Read the model definition and answer for the solid it produces. Units are mm, in the model's axes. Face numbers are marked on the shaded views. Round coordinates to 2 decimals unless told otherwise and drop trailing zeros. Write each loop counter-clockwise with the first axis right and the second up, starting at its lowest first coordinate (ties: lowest second). Pieces come first, ordered by that corner, then holes. Notation, with made-up numbers: (33.5, 29.5) -> (39.5, 29.5) arc R19 cw to (39.5, 45.5) -> close; hole circle Ø5 at (48, 27.5). An arc over 180 degrees is marked (long way). Return JSON: item names as keys, results as strings.
from build123d import *

# Parameters (mm, degrees)
BOSS_EXTRUDE1_DEPTH = 6.35
SKETCH2_W           = 18
SKETCH2_H           = 6.35
CUT_EXTRUDE1_DEPTH  = 148.509567486
SKETCH4_W           = 60
SKETCH4_H           = 105
CUT_EXTRUDE2_DEPTH  = 3.1
SKETCH5_R           = 1.6
CUT_EXTRUDE3_DEPTH  = 148.509567486


with BuildPart() as part:
    # Sketch1 → Boss-Extrude1 (new body)
    with BuildSketch(Plane(origin=(0, 0, 0), x_dir=(1, 0, 0), z_dir=(0, 1, 0))):
        Polygon((64.951905284, 87.5), (-64.951905284, 87.5), (-108.253175473, 12.5), (-43.301270189, -100), (43.301270189, -100), (108.253175473, 12.5), align=None)
    extrude(amount=BOSS_EXTRUDE1_DEPTH)

    # Sketch2 → Cut-Extrude1 (cut, through all)
    with BuildSketch(Plane(origin=(0, 6.35, 0), x_dir=(1, 0, 0), z_dir=(0, 1, 0))):
        with Locations((-29, -90.525)):
            Rectangle(SKETCH2_W, SKETCH2_H)
        with Locations((29, -90.525)):
            Rectangle(SKETCH2_W, SKETCH2_H)
        Polygon((-62.146580335, 79.758965344), (-56.647319021, 76.583965344), (-65.647319021, 60.995508076), (-71.146580335, 64.170508076), align=None)
        Polygon((-94.647319021, 10.766034656), (-85.647319021, 26.354491924), (-91.146580335, 29.529491924), (-100.146580335, 13.941034656), align=None)
        Polygon((100.146580335, 13.941034656), (91.146580335, 29.529491924), (85.647319021, 26.354491924), (94.647319021, 10.766034656), align=None)
        Polygon((56.647319021, 76.583965344), (62.146580335, 79.758965344), (71.146580335, 64.170508076), (65.647319021, 60.995508076), align=None)
    extrude(amount=-CUT_EXTRUDE1_DEPTH, mode=Mode.SUBTRACT)

    # Sketch4 → Cut-Extrude2 (cut)
    with BuildSketch(Plane(origin=(0, 6.35, 0), x_dir=(1, 0, 0), z_dir=(0, 1, 0))):
        Rectangle(SKETCH4_W, SKETCH4_H)
    extrude(amount=-CUT_EXTRUDE2_DEPTH, mode=Mode.SUBTRACT)

    # Sketch5 → Cut-Extrude3 (cut, through all)
    with BuildSketch(Plane(origin=(0, 6.35, 0), x_dir=(1, 0, 0), z_dir=(0, 1, 0))):
        with Locations(Location((0, 72.5, 0), (0, 0, 270))):
            Circle(SKETCH5_R)
        with Locations(Location((-62.786841774, -36.25, 0), (0, 0, 270))):
            Circle(SKETCH5_R)
        with Locations(Location((62.786841774, -36.25, 0), (0, 0, 270))):
            Circle(SKETCH5_R)
    extrude(amount=-CUT_EXTRUDE3_DEPTH, mode=Mode.SUBTRACT)


solid = part.part
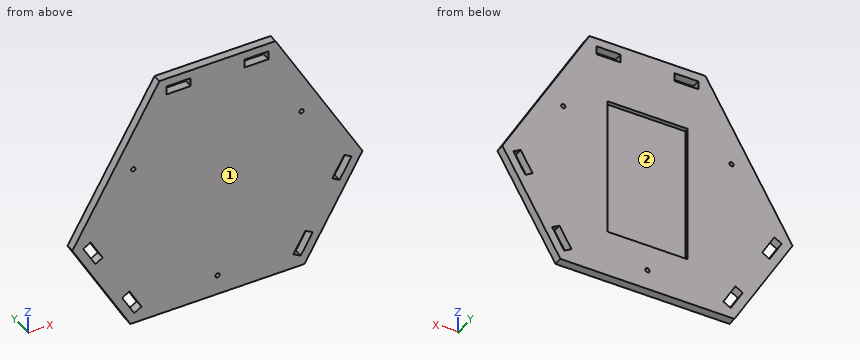
Item 1: Section C-C (z = 49) is taken. Give the vertices of the cut face in (x, y), then the cut area to 3 significant figures.
Worked answers:
{"outline": "(-72.75, 0) -> (72.75, 0) -> (72.75, 6.35) -> (30, 6.35) -> (30, 3.25) -> (-30, 3.25) -> (-30, 6.35) -> (-72.75, 6.35) -> close", "area": "738 mm2"}
Item 2: Section A-A (z = -23.5) is taken. Give the vertices of the cut face in (x, y).
Worked answers:
{"outline": "(-101.9, 0) -> (-94.63, 0) -> (-94.63, 6.35) -> (-101.9, 6.35) -> close; (-87.3, 0) -> (87.3, 0) -> (87.3, 6.35) -> (30, 6.35) -> (30, 3.25) -> (-30, 3.25) -> (-30, 6.35) -> (-87.3, 6.35) -> close; (94.63, 0) -> (101.9, 0) -> (101.9, 6.35) -> (94.63, 6.35) -> close"}
Item 3: Section D-D (x = 80) is taken. Give the vertices of the cut face in (y, z).
Worked answers:
{"outline": "(0, -61.44) -> (6.35, -61.44) -> (6.35, 36.44) -> (0, 36.44) -> close"}
Item 4: For a pull along X with two mould halves and no side action, classify the marked faces 1 and 2 as released by +X, released by -X, zero draft, split by the parting line, or undercut.
Worked answers:
{"face 1": "zero draft", "face 2": "undercut"}
Item 5: Section B-B (y = 4.75) is taken. State how many separate pieces and enclosed holes the cut face has, then the cut area to 3 significant figures.
Worked answers:
{"separate pieces": "1", "enclosed holes": "10", "area": "23,000 mm2"}
Item 6: Straight lines are drawn through the part: L1, parallel to Z at x = -34.5, y = 5.25; L2, parallel to X at y = 2.5, z = 36.25; L3, parallel to X at y = 4.5, z = 36.25. For each, find the intervals that lie inside material, in ascending order. Write a range as [from, to].
Worked answers:
{"L1": "z = [-87.5, 87.35], [93.7, 100]", "L2": "x = [-80.11, -64.39], [-61.19, 61.19], [64.39, 80.11]", "L3": "x = [-80.11, -64.39], [-61.19, -30], [30, 61.19], [64.39, 80.11]"}
Item 7: Flat-ended cylindrical pins translate along their axes: pin 1 (1.9 mm diameter, centred on y = 2.5, z = 92, fed in from +X); pin 2 (3 mm diameter, centred on y = 3, z = 90.5, fed in from -X); pin 3 (3.5 mm diameter, centred on y = 5, z = -9, fed in from -X). Find the tip coordinate at first contact, or state that the pin passes through.
Worked answers:
{"pin 1": "stops at x = 48.47", "pin 2": "stops at x = -49.65", "pin 3": "stops at x = -107.24"}
